For this review, take the finished solid that the model builds, in its own axes (mm). Give positions to 0.01 mm unless a question says otherwise; leave off trailing zeros. Loops run counter-clockwise (first coordinate to the right, second up) from the corner with the lowest first, then second, coordinate; pieces in that order, holes last. Notation, with made-up numbers: (39, 39) - (85, 39) arc R17 cw to (85, 72) - close; hole circle Ø3 at (53.25, -21.5). An arc over 180 degrees is marked (long way). Use CSV: the item, a comma, the result in double quotes. Start each with the question number.
1. Take a section at A-A on x = 0. Give the boundary of the cut face in (y, z), plus the area to 3 significant figures.
2. Take a section at C-C on y = 19. Give the boundary of the cut face in (x, z), plus the area to 3 significant figures.
3. Take a section at B-B on z = 1.75. Give the boundary of the cut face in (x, y), plus the area to 3 significant figures.
4. Wall thickness on line 1 (Y direction, x = 0, z = 8.5); line 2 (Y direction, x = -1.25, z = 8); line 3 (X direction, y = 48.5, z = 9.5): over which ranges is each line inside the solid? List them lowest first.
5. Take a section at D-D on z = 10.5. Give the boundary of the cut face in (x, y), plus the area to 3 significant figures.
6. For pin 1 (0.8 mm diameter, centred on x = -0.5, y = 49.5, fed in from +Z); pin 2 (1.5 mm diameter, centred on y = 42, z = -2.5, fed in from -X), all flat-tipped, find the tip position at first contact; note any pin that passes through.
```python
from build123d import *

# Parameters (mm, degrees)
SKETCH1_R           = 2.55
BOSS_EXTRUDE1_DEPTH = 58
SKETCH2_R           = 1.4
CUT_EXTRUDE1_DEPTH  = 10


with BuildPart() as part:
    # Sketch1 → Boss-Extrude1 (new body)
    with BuildSketch(Plane(origin=(0, 0, 0), x_dir=(1, 0, 0), z_dir=(0, 1, 0))):
        with BuildLine():
            Line((-5.75, 0), (-5.75, -15))
            Line((-5.75, -15), (5.75, -15))
            Line((5.75, -15), (5.75, 0))
            ThreePointArc((5.75, 0), (0, 5.75), (-5.75, 0))
        make_face()
        with Locations(Location((0, 0, 0), (0, 0, 90))):
            Circle(SKETCH1_R, mode=Mode.SUBTRACT)
    extrude(amount=BOSS_EXTRUDE1_DEPTH)

    # Sketch2 → Cut-Extrude1 (cut)
    with BuildSketch(Plane.XY.offset(15)):
        with Locations((0, 49)):
            Circle(SKETCH2_R)
        with Locations((0, 39)):
            Circle(SKETCH2_R)
        with Locations((0, 29)):
            Circle(SKETCH2_R)
        with Locations((0, 19)):
            Circle(SKETCH2_R)
        with Locations((0, 9)):
            Circle(SKETCH2_R)
    extrude(amount=-CUT_EXTRUDE1_DEPTH, mode=Mode.SUBTRACT)


solid = part.part
```
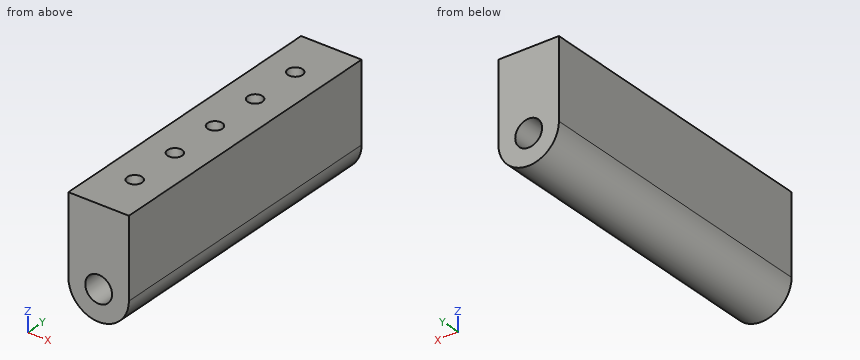
Check result:
1,outline,"(0, -5.75) - (58, -5.75) - (58, -2.55) - (0, -2.55) - close; (0, 2.55) - (58, 2.55) - (58, 15) - (50.4, 15) - (50.4, 5) - (47.6, 5) - (47.6, 15) - (40.4, 15) - (40.4, 5) - (37.6, 5) - (37.6, 15) - (30.4, 15) - (30.4, 5) - (27.6, 5) - (27.6, 15) - (20.4, 15) - (20.4, 5) - (17.6, 5) - (17.6, 15) - (10.4, 15) - (10.4, 5) - (7.6, 5) - (7.6, 15) - (0, 15) - close"
1,area,"768 mm²"
2,outline,"(-5.75, 0) arc R5.75 ccw to (5.75, 0) - (5.75, 15) - (1.4, 15) - (1.4, 5) - (-1.4, 5) - (-1.4, 15) - (-5.75, 15) - close; hole circle Ø5.1 at (0, 0)"
2,area,"176 mm²"
3,outline,"(-5.75, 0) - (-1.85, 0) - (-1.85, 58) - (-5.75, 58) - close; (1.85, 0) - (5.75, 0) - (5.75, 58) - (1.85, 58) - close"
3,area,"452 mm²"
4,line 1,"y = 0 to 7.6, 10.4 to 17.6, 20.4 to 27.6, 30.4 to 37.6, 40.4 to 47.6, 50.4 to 58"
4,line 2,"y = 0 to 8.37, 9.63 to 18.37, 19.63 to 28.37, 29.63 to 38.37, 39.63 to 48.37, 49.63 to 58"
4,line 3,"x = -5.75 to -1.31, 1.31 to 5.75"
5,outline,"(-5.75, 0) - (5.75, 0) - (5.75, 58) - (-5.75, 58) - close; hole circle Ø2.8 at (0, 9); hole circle Ø2.8 at (0, 19); hole circle Ø2.8 at (0, 29); hole circle Ø2.8 at (0, 39); hole circle Ø2.8 at (0, 49)"
5,area,"636 mm²"
6,pin 1,"stops at z = 5"
6,pin 2,"stops at x = -5.48"
